from build123d import *

# Parameters (mm, degrees)
F0_R     = 6
F0_R_2   = 1.6
F0_W     = 35
F0_H     = 3.2
F1_DEPTH = 2.4
F2_SIZE  = 0.4
F3_R     = 30
F4_R     = 5


with BuildPart() as f1:
    # F0 (on Top) → F1 (new body)
    with BuildSketch(Plane.XY):
        with BuildLine():
            Line((-8.000963252, 2.3046399066), (-8, -40.4145188433))
            ThreePointArc((-8, -40.4145188433), (0, -48.4145188433), (8, -40.4145188433))
            Line((8, -40.4145188433), (7.9974217916, 2.303660399))
            Line((7.9974217916, 2.303660399), (37.6375477343, 12.6545551411))
            ThreePointArc((37.6375477343, 12.6545551411), (42.6856959969, 22.427637102), (33.2034437111, 28.002923954))
            Line((33.2034437111, 28.002923954), (-0.0031576851, 20.3502692862))
            Line((-0.0031576851, 20.3502692862), (-33.2031192071, 28.002849163))
            ThreePointArc((-33.2031192071, 28.002849163), (-42.6856411927, 22.4278267944), (-37.6376061638, 12.654575546))
            Line((-37.6376061638, 12.654575546), (-8.000963252, 2.3046399066))
        make_face()
        with Locations((0, -40.4145188433)):
            Circle(F0_R, mode=Mode.SUBTRACT)
        with Locations((0, -14.8963702892)):
            Circle(F0_R_2, mode=Mode.SUBTRACT)
        with Locations((-35, 20.2072594216)):
            Circle(F0_R, mode=Mode.SUBTRACT)
        with Locations((0, 10.1036297108)):
            Rectangle(F0_W, F0_H, mode=Mode.SUBTRACT)
        with Locations((35, 20.2072594216)):
            Circle(F0_R, mode=Mode.SUBTRACT)
    extrude(amount=F1_DEPTH)

    # F2
    f2_edges = [f1.edges().sort_by_distance(p)[0] for p in [
        (-17.5, 10.10363, 2.4),
        (0, 11.70363, 2.4),
        (0, 8.50363, 2.4),
        (17.5, 10.10363, 2.4),
    ]]
    chamfer(f2_edges, length=F2_SIZE)

    # F3
    f3_edges = [f1.edges().sort_by_distance(p)[0] for p in [
        (-0.003158, 20.350269, 1.2),
    ]]
    fillet(f3_edges, radius=F3_R)

    # F4
    f4_edges = [f1.edges().sort_by_distance(p)[0] for p in [
        (7.997422, 2.30366, 1.2),
        (-8.000963, 2.30464, 1.2),
    ]]
    fillet(f4_edges, radius=F4_R)


solid = f1.part
Verification items for the finished model (mm, model axes). A direction names the side the tool comes from. Give positions to 0.01 mm unless a question says otherwise; leave off trailing zeros. Loops run counter-clockwise (first coordinate to the right, second up) from the corner with the lowest first, then second, coordinate; pieces in that order, holes last. Notation, with made-up numbers: (12, 34) - (26, 34) arc R22 ccw to (26, 53) - close; hole circle Ø7 at (-16, -19.75). An arc over 180 degrees is marked (long way). Write item = value, one per line. Start each with the question number.
Q1. Thickness scan on line 1 (Y direction, x = 0, z = 0.7); line 2 (Y direction, x = -5, z = 0.1); line 3 (X direction, y = -34, z = 1.9). Record the ranges inside material, lowest first.
Q2. Depth check by flat-ended pin: P1, Ø1.2, axis at y = -26.5, z = 1.5, coming from the -X side; P2, Ø0.6, axis at x = 1, z = 1.5, coming from the -Y side. Enter the tip coordinate at first touch or a pass-through.
Q3. Cross-section at A-A, the plane x = 0. Enter the section's corners in (y, z), and give its area (3 significant figures).
Q4. Cross-section at C-C, the plane x = -13.5. Enter the section's corners in (y, z).
Q5. Mould release check, pull along X, two halves, no side actions. Record for faces 4 (the face through (-0.098, 21.137, 1.217)), 5 (the face through (-0.176, -48.413, 1.183)), 6 (the face through (0, 4, 2.4)): released by +X, released by -X, zero draft, split by the parting line, or undercut.
Q6. Tool access check on faces 1 (the face through (-19.79, 24.91, 1.18)), 2 (the face through (0, 8.504, 1)), 3 (the face through (24.31, 8, 1.18)). Record the directions out of +Z, -Z, +X, -X, +Y, -Y that give a thin tool (end or side, any length) a straight path to the whole face; none if there is none.
Q7. Cross-section at D-D, the plane x = -35. Enter the section's corners in (y, z).
Q8. Cross-section at B-B, the plane y = -35.5. Enter the section's corners in (x, z).
Answer key:
q1.line_1 = -48.41 to -46.41, -34.41 to -16.5, -13.3 to 8.5, 11.7 to 21.14
q1.line_2 = -46.66 to -43.73, -37.1 to 8.5, 11.7 to 21.56
q1.line_3 = -8 to 8
q2.P1 = -8
q2.P2 = -48.38
q3.outline = (-48.41, 0) - (-46.41, 0) - (-46.41, 2.4) - (-48.41, 2.4) - close; (-34.41, 0) - (-16.5, 0) - (-16.5, 2.4) - (-34.41, 2.4) - close; (-13.3, 0) - (8.5, 0) - (8.5, 2) - (8.1, 2.4) - (-13.3, 2.4) - close; (11.7, 0) - (21.14, 0) - (21.14, 2.4) - (12.1, 2.4) - (11.7, 2) - close
q3.area = 123 mm^2
q4.outline = (4.23, 0) - (8.5, 0) - (8.5, 2) - (8.1, 2.4) - (4.23, 2.4) - close; (11.7, 0) - (23.46, 0) - (23.46, 2.4) - (12.1, 2.4) - (11.7, 2) - close
q5.face_4 = undercut
q5.face_5 = split by the parting line
q5.face_6 = zero draft
q6.face_1 = +Z, -Z, +Y
q6.face_2 = +Z, -Z
q6.face_3 = +Z, -Z, +X, -Y
q7.outline = (11.73, 0) - (14.21, 0) - (14.21, 2.4) - (11.73, 2.4) - close; (26.21, 0) - (28.21, 0) - (28.21, 2.4) - (26.21, 2.4) - close
q8.outline = (-8, 0) - (-3.44, 0) - (-3.44, 2.4) - (-8, 2.4) - close; (3.44, 0) - (8, 0) - (8, 2.4) - (3.44, 2.4) - close
